Check sheet for the modelled part. Datum: model origin and axes. Units: mm. A direction names the side the tool comes from. Round coordinates to 2 decimals unless told otherwise and drop trailing zeros. Order: outer loops, then holes, each group sorted by start corner. A loop starts at its lowest first (then second) coordinate and runs counter-clockwise, first axis right, second up.
```python
from build123d import *

# Parameters (mm, degrees)
F0_R     = 10.95
F1_DEPTH = 3
F2_R     = 3.95
F3_DEPTH = 6.9
F4_T     = -2


# Not quite as in the source:
# - a fillet or chamfer that OpenCascade refuses, or shapes differently, is made with other operations: its cross-section is extruded or revolved along the edge and cut away or added


with BuildPart() as f1:
    # F0 (on Front) → F1 (new body)
    with BuildSketch(Plane.XZ):
        Circle(F0_R)
    extrude(amount=F1_DEPTH)

    # F2 (on Front) → F3 (join)
    with BuildSketch(Plane.XZ):
        Circle(F2_R)
    extrude(amount=F3_DEPTH)

    # F4
    f4_openings = [f1.faces().sort_by_distance(p)[0] for p in [
        (0, -6.9, 0),
    ]]
    offset(amount=F4_T, openings=f4_openings, kind=Kind.INTERSECTION)

    # F5: fillet of radius 3.81 on 1 edges, made by hand

    # F5_s1 → F5_t2 (revolve, cut)
    with BuildSketch(Plane.XY):
        with BuildLine():
            ThreePointArc((10.95, -3), (9.6177045238, -0.843335206), (7.2270979062, 0))
            Line((7.2270979062, 0), (10.95, 0))
            Line((10.95, 0), (10.95, -3))
        make_face()
    revolve(axis=Axis((0, 0, 0), (0, -1, 0)), mode=Mode.SUBTRACT)


solid = f1.part
```
Item 1: Sectioned sample at D-D (y = -2.5). Record the cut outline in (x, z).
Answer:
outline: circle Ø21.61 at (0, 0); hole circle Ø3.9 at (0, 0)
Item 2: Sectioned sample at B-B (x = 0). Record the cut outline in (y, z).
Answer:
outline: (-6.9, -3.95) - (-3, -3.95) - (-3, -10.95) arc R3.81 ccw to (0, -7.23) - (0, 7.23) arc R3.81 ccw to (-3, 10.95) - (-3, 3.95) - (-6.9, 3.95) - (-6.9, 1.95) - (-2, 1.95) - (-2, -1.95) - (-6.9, -1.95) - close
Item 3: Scan lines: line 1 along Z through (x, y) = (0, -4.95); line 2 along Y through (x, z) = (2, 6.5). Record each from-to range of solid material in increasing order.
Answer:
line 1: z = -3.95 to -1.95, 1.95 to 3.95
line 2: y = -3 to 0
Item 4: Sectioned sample at A-A (z = 0). Record the cut outline in (x, y), and give its area (3 significant figures).
Answer:
outline: (-10.95, -3) - (-3.95, -3) - (-3.95, -6.9) - (-1.95, -6.9) - (-1.95, -2) - (1.95, -2) - (1.95, -6.9) - (3.95, -6.9) - (3.95, -3) - (10.95, -3) arc R3.81 ccw to (7.23, 0) - (-7.23, 0) arc R3.81 ccw to start
area: 71.7 mm2
Item 5: Sectioned sample at C-C (y = -4.75). Record the cut outline in (x, z).
Answer:
outline: circle Ø7.9 at (0, 0); hole circle Ø3.9 at (0, 0)
Item 6: Go/stop test with flat-tipped pins: P1, Ø4, axis at x = -4, y = -2, coming from the +Z side; P2, Ø2, axis at y = -1, z = -4, coming from the -X side; P3, Ø3, axis at x = 1.5, z = -6, coming from the -Y side; P4, Ø1.5, axis at x = 8.5, y = -5, coming from the +Z side. Record where each tip stops, or that it passes through.
Answer:
P1: stops at z = 10.71
P2: stops at x = -9.9
P3: stops at y = -3
P4: passes through
Item 7: Release check for a two-part mould opening along X. For faces 1 (the flat face through (0, 0, 0)), 2 (the cylindrical face through (-3.135, -4.923, -2.404)), 3 (the flat face through (0, -2, 0)) record: released by +X, released by -X, zero draft, split by the parting line, or undercut.
Answer:
face 1: zero draft
face 2: split by the parting line
face 3: undercut
Item 8: Access from +Z, -Z, +X, -X, +Y, -Y to the whole of each face (thin tool, end or side, straight path). Record for faces 4 (the cylindrical face through (-0.254, -4.416, 1.933)), 5 (the flat face through (-2, -6.9, -1)).
Answer:
face 4: -Y
face 5: +Z, -Z, +X, -X, -Y
